```python
from build123d import *

# Parameters (mm, degrees)
SKETCH1_W           = 25.4
SKETCH1_H           = 50.8
SKETCH1_W_2         = 19.05
SKETCH1_H_2         = 44.45
BOSS_EXTRUDE1_DEPTH = 279.4
CUT_EXTRUDE1_REACH  = 287.114
SKETCH2_W           = 50.8
SKETCH2_H           = 25.4


with BuildPart() as part:
    # Sketch1 → Boss-Extrude1 (new body)
    with BuildSketch(Plane.XY):
        with Locations((12.7, -25.4)):
            Rectangle(SKETCH1_W, SKETCH1_H)
        with Locations((12.7, -25.4)):
            Rectangle(SKETCH1_W_2, SKETCH1_H_2, mode=Mode.SUBTRACT)
    extrude(amount=BOSS_EXTRUDE1_DEPTH)

    # Cut-Extrude1: up to this face of the body (flat: up to its plane)
    cut_extrude1_end = Plane(part.part.faces().sort_by_distance((0, -25.4, 139.7))[0])
    # Sketch2 → Cut-Extrude1 (cut, up to the picked face)
    with BuildSketch(Plane(origin=(25.4, 0, 0), x_dir=(0, 0, -1), z_dir=(1, 0, 0)), mode=Mode.PRIVATE) as cut_extrude1_sk1:
        with Locations((-254, -12.7)):
            Rectangle(SKETCH2_W, SKETCH2_H)
    cut_extrude1_tool1 = split(extrude(cut_extrude1_sk1.sketch, amount=-CUT_EXTRUDE1_REACH, mode=Mode.PRIVATE), bisect_by=cut_extrude1_end, keep=Keep.BOTH, mode=Mode.PRIVATE)
    add(cut_extrude1_tool1.solids().sort_by(Axis((25.4, -12.7, 254), (-1, 0, 0)))[0], mode=Mode.SUBTRACT)


solid = part.part
```
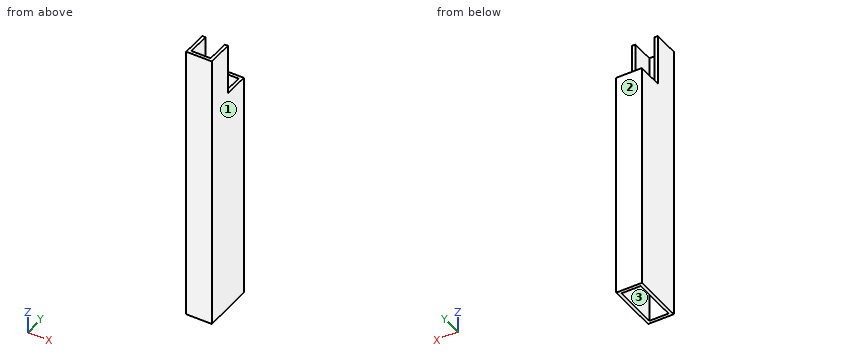
CAD build for the part. Positions are in the model's coordinates, mm. Face numbers are marked on the shaded views. Give positions to 0.01 mm unless a question says otherwise; leave off trailing zeros. Order: outer loops, then holes, each group sorted by start corner. A loop starts at its lowest first (then second) coordinate and runs counter-clockwise, first axis right, second up.
(1) Flat gauge pins, fed straight in: pin 1 (1.5 mm diameter, centred on x = 2.5, z = 125.5, fed in from +Y); pin 2 (1 mm diameter, centred on x = 20.5, y = -32, fed in from +Z); pin 3 (1.6 mm diameter, centred on x = 24.5, z = 261.5, fed in from +Y). Where does each tip first touch, or does it go through?
(2) Saw through at A-A, the plane x = 14.75. Give the cut face in (y, z) (3 decimals).
(3) Saw through at C-C, the plane z = 43. Give the cut face in (x, y) (3 decimals), then the cut area to 3 significant figures.
(4) Saw through at B-B, the plane y = -14.5. Give the cut face in (x, z) (3 decimals), then the cut area to 3 significant figures.
(5) Mould opens along Y. For the marked faces 1, 2 and 3 say: released by +Y, released by -Y, zero draft, split by the parting line, or undercut.
(6) Saw through at D-D, the plane z = 251. Give the cut face in (x, y) (3 decimals).
(7) Drill centre lines: L1, parallel to X at y = -4, z = 91 (3 decimals); L2, parallel to Y at x = 11.25, z = 56.5 (3 decimals); L3, parallel to Y at x = 16.5, z = 231 (3 decimals). Where is each one in solid material? Low to high.
Results found:
1. pin 1: stops at y = 0
1. pin 2: passes through
1. pin 3: stops at y = -25.4
2. outline: (-50.8, 0) - (-47.625, 0) - (-47.625, 279.4) - (-50.8, 279.4) - close; (-3.175, 0) - (0, 0) - (0, 228.6) - (-3.175, 228.6) - close
3. outline: (0, -50.8) - (25.4, -50.8) - (25.4, 0) - (0, 0) - close; hole (3.175, -47.625) - (22.225, -47.625) - (22.225, -3.175) - (3.175, -3.175) - close
3. area: 444 mm2
4. outline: (0, 0) - (3.175, 0) - (3.175, 228.6) - (0, 228.6) - close; (22.225, 0) - (25.4, 0) - (25.4, 228.6) - (22.225, 228.6) - close
4. area: 1,450 mm2
5. face 1: zero draft
5. face 2: released by +Y
5. face 3: undercut
6. outline: (0, -50.8) - (25.4, -50.8) - (25.4, -25.4) - (22.225, -25.4) - (22.225, -47.625) - (3.175, -47.625) - (3.175, -25.4) - (0, -25.4) - close
7. L1: x = 0 to 3.175, 22.225 to 25.4
7. L2: y = -50.8 to -47.625, -3.175 to 0
7. L3: y = -50.8 to -47.625
